Answer from the drawing. Dimensions are ordinates in mm from the lowest x, y and z of the part. Give positions to 0.01 mm unless a question says otherwise; leave off trailing zeros. Write each loop counter-clockwise with the first axis right and the second up, starting at its lowest first coordinate (ties: lowest second). Pieces come first, ordered by that corner, then holes.
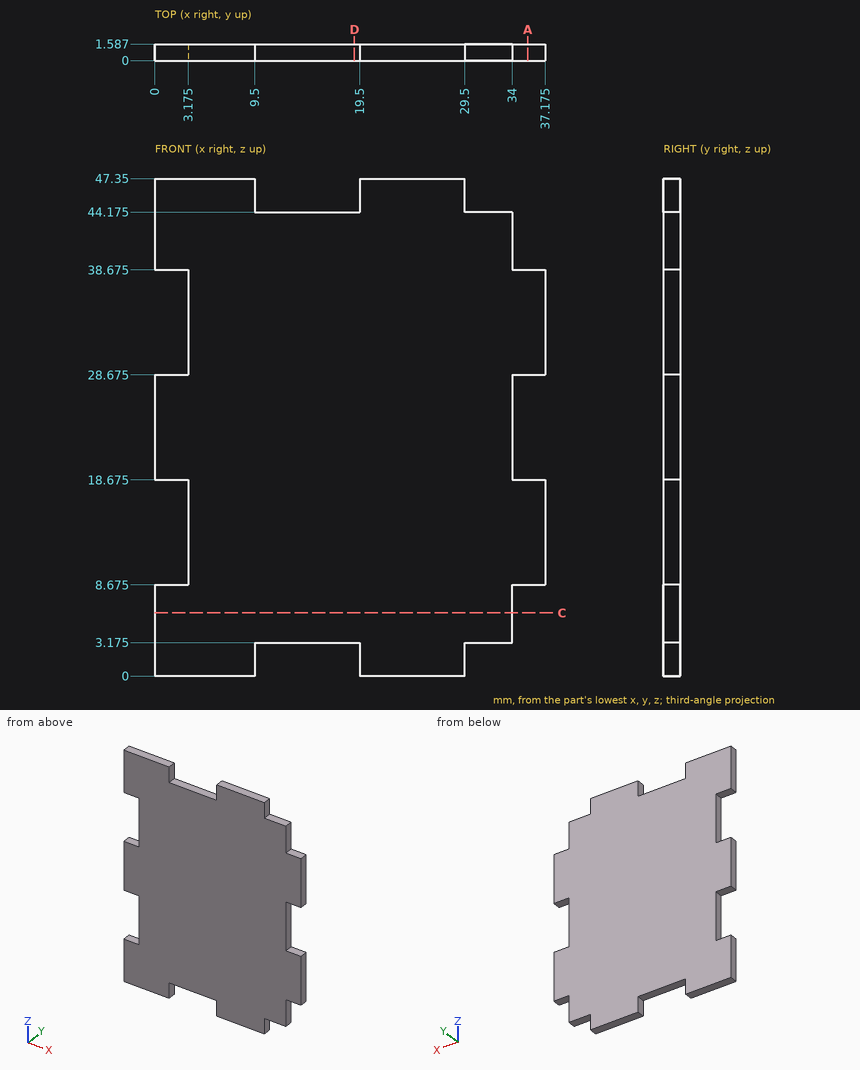
Item 1: Section C-C (z = 6) is taken. Write down the section's boundary in (x, y).
Result set:
outline: (0, 0) - (34, 0) - (34, 1.59) - (0, 1.59) - close
Item 2: Section D-D (x = 19) is taken. Write down the section's boundary in (y, z) (1 decimal).
Result set:
outline: (0, 3.2) - (1.6, 3.2) - (1.6, 44.2) - (0, 44.2) - close
Item 3: This flat-tipped pin is pushed along its axis until it touches: pin 1 Ø0.8 at (x, y) = (30.5, 0.5) entering from +Z (1 decimal). Where does it stop, or does it pass through?
Result set:
pin 1: stops at z = 44.2
Item 4: Section A-A (x = 35.5) is taken. Write down the section's boundary in (y, z) (1 decimal).
Result set:
outline: (0, 8.7) - (1.6, 8.7) - (1.6, 18.7) - (0, 18.7) - close; (0, 28.7) - (1.6, 28.7) - (1.6, 38.7) - (0, 38.7) - close
Item 5: Find the intervals of material crossed by line 1 along X through (y, z) = (0.6, 12.5) (1 decimal); line 2 along Z through (x, y) = (11, 1) (1 decimal); line 3 along X through (y, z) = (0.3, 40), in increasing order.
Result set:
line 1: x = 3.2 to 37.2
line 2: z = 3.2 to 44.2
line 3: x = 0 to 34
